```python
from build123d import *

# Parameters (mm, degrees)
F2_R   = 8.65
F2_R_2 = 6.35


with BuildPart() as f1:
    # F0 (on Front) → F1 (revolve)
    with BuildSketch(Plane.XZ):
        Polygon((6.35, 6.4351068075), (6.35, 0), (8.65, 0), (18.5, 3.5851068075), (18.5, 6.4351068075), align=None)
    revolve(axis=Axis((0, 0, 5.6449943222), (0, 0, 1)))

    # F4: sweep along a path in F3
    with BuildLine(Plane.YZ) as f4_path:
        Line((0, 0), (0, -120))
        ThreePointArc((0, -120), (8.7867965644, -141.2132034356), (30, -150))
        Line((30, -150), (100, -150))
    # F2 (on Top) → F4 (sweep)
    with BuildSketch(Plane.XY):
        Circle(F2_R)
        Circle(F2_R_2, mode=Mode.SUBTRACT)
    sweep(path=f4_path.line)


solid = f1.part
```
Read the model definition and answer for the solid it produces. Units are mm, in the model's axes. A direction names the side the tool comes from. Give positions to 0.01 mm unless a question says otherwise; leave off trailing zeros. Order: outer loops, then holes, each group sorted by start corner. A loop starts at its lowest first (then second) coordinate and runs counter-clockwise, first axis right, second up. Notation, with made-up numbers: (-36, 54) -> (-21, 54) arc R31 ccw to (-21, 80) -> close; hole circle Ø8 at (4.5, 18.5). An arc over 180 degrees is marked (long way). One line per item, written item: value. Start each with the question number.
(1) The part is cut by section A-A (x = 0). Determine the outline of the cut face in (y, z), and give its area (3 significant figures).
(2) A tool of negligible diameter and unlimited length cuts with its end or side. For faces 1 (the cylindrical face through (-1.38, -6.2, -57.67)), 2 (the flat face through (8, 0, 6.435)), 3 (the cylindrical face through (-1.126, 65.49, -158.576)), 4 (the cylindrical face through (8.25, -2.6, -60.84)), from which of +Z, -Z, +X, -X, +Y, -Y can it reach the whole face along a straight path? Write none if from no direction.
(3) For a pull along X with two mould halves and no side action, classify faces 5 (the cylindrical face through (-0.8, 65.5, -156.3)), 6 (the flat face through (6, 100, -147)), 7 (the conical face through (4.981, 7.813, 0.224)) as released by +X, released by -X, zero draft, split by the parting line, or undercut.
(4) The part is cut by section C-C (y = 53). Determine the outline of the cut face in (x, z).
(5) Flat-ended cylindrical pins translate along their axes: P1, Ø6, axis at x = 1.5, z = -32, coming from the +Y side; P2, Ø3, axis at y = 3, z = -122, coming from the -X side; P3, Ø20.5, axis at x = 0, z = -150, coming from the -Y side. Find the tip coordinate at first contact, or state that the pin passes through.
(6) Straight lines are drawn through the part: L1, parallel to Y at x = 0, z = -74; L2, parallel to Z at x = 1, y = 15. For each, find the intervals that lie inside material, in ascending order.
(7) The part is cut by section B-B (z = -101.5). Determine the outline of the cut face in (x, y), and give its area (3 significant figures).
Taken from the geometry:
1. outline: (-18.5, 3.59) -> (-8.65, 0) -> (-8.65, -120) arc R38.65 ccw to (30, -158.65) -> (100, -158.65) -> (100, -156.35) -> (30, -156.35) arc R36.35 cw to (-6.35, -120) -> (-6.35, 6.44) -> (-18.5, 6.44) -> close; (6.35, -120) arc R23.65 ccw to (30, -143.65) -> (100, -143.65) -> (100, -141.35) -> (30, -141.35) arc R21.35 cw to (8.65, -120) -> (8.65, 0) -> (18.5, 3.59) -> (18.5, 6.44) -> (6.35, 6.44) -> close
1. area: 1,210 mm^2
2. face 1: +Z
2. face 2: +Z, +X, -X, +Y, -Y
2. face 3: +Y
2. face 4: none
3. face 5: undercut
3. face 6: zero draft
3. face 7: split by the parting line
4. outline: circle Ø17.3 at (0, -150); hole circle Ø12.7 at (0, -150)
5. P1: y = 8.65
5. P2: x = -8.53
5. P3: y = -3.22
6. L1: -8.65 to -6.35, 6.35 to 8.65
6. L2: -155.56 to -153.02, -138.39 to -135.27, 2.32 to 6.44
7. outline: circle Ø17.3 at (0, 0); hole circle Ø12.7 at (0, 0)
7. area: 108 mm^2
